Can you work these out from the model? Positions are in its coordinate system, mm. A direction names the side the tool comes from. Give positions to 0.01 mm unless a question says otherwise; leave off trailing zeros. Order: outer loops, then holes, each group sorted by start corner. A loop starts at its lowest first (then second) coordinate and runs counter-clockwise, first axis right, second up. Notation, with made-up numbers: (-29, 18) - (-5, 18) arc R21 cw to (-5, 40) - close; hole circle Ø3 at (16, 89.5). An arc over 180 degrees is marked (long way). Use one line per item in the form item = value. Start each with the question number.
1) Suppose I cut it at D-D, the plane z = 34.5. Write out the boundary of the cut face in (x, y).
2) Which directions (+Z, -Z, +X, -X, +Y, -Y) give clear straight access to the entire face, cutting with the end or side of a thin tool? Please do faces 5 (the flat face through (3, -1, 14)), 6 (the flat face through (7, 30, 1)), 7 (the flat face through (14, 0, 26)), 8 (the flat face through (14, -2, 1)), 9 (the flat face through (15, -22, 36)).
3) Suppose I cut it at C-C, the plane x = 5.25. Write out the boundary of the cut face in (y, z).
4) Please list where these lines run through material, in increasing order: probe 1 along Y at (x, z) = (24.75, 1.1); probe 2 along X at (y, z) = (-1, 23); probe 3 along Y at (x, z) = (26.25, 36).
5) We'd pull the mould along Z, two halves only. Please class faces 1 (the flat face through (15, 19, 0)), 2 (the flat face through (23, 30, 1)), 3 (the flat face through (15, -21, 47)), 4 (the cylindrical face through (9.1, -21, 35.7)): released by +Z, released by -Z, zero draft, split by the parting line, or undercut.
6) Suppose I cut it at A-A, the plane x = 10. Write out the boundary of the cut face in (y, z), and give its area (4 significant figures).
7) For pin 1 (1.8 mm diameter, centred on x = 20, z = 34.5, fed in from +Y); pin 2 (4 mm diameter, centred on x = 9, y = 5, fed in from +Z); pin 3 (17.5 mm diameter, centred on x = 12, y = -12.5, fed in from -Z); pin 4 (0.6 mm diameter, centred on x = 17, z = 1.5, fed in from -Y), each with a flat end and sliding along its axis, tell me the tip position at first contact or that it passes through.
8) Suppose I cut it at B-B, the plane z = 9. Write out the boundary of the cut face in (x, y), and give its area (3 significant figures).
```python
from build123d import *

# Parameters (mm, degrees)
SKETCH1_W           = 30
SKETCH1_H           = 40
BOSS_EXTRUDE1_DEPTH = 2
BOSS_EXTRUDE3_DEPTH = 30
SKETCH6_W           = 24
SKETCH6_H           = 23
CUT_EXTRUDE2_DEPTH  = 2
SKETCH7_R           = 1.5
SKETCH7_W           = 16
SKETCH7_H           = 2.75
CUT_EXTRUDE3_DEPTH  = 10
SKETCH9_R           = 1.5
CUT_EXTRUDE4_DEPTH  = 10


with BuildPart() as part:
    # Sketch1 → Boss-Extrude1 (new body)
    with BuildSketch(Plane.XY):
        with Locations((15, 20)):
            Rectangle(SKETCH1_W, SKETCH1_H)
    extrude(amount=BOSS_EXTRUDE1_DEPTH)

    # Sketch5 → Boss-Extrude3 (add)
    with BuildSketch(Plane(origin=(0, 0, 0), x_dir=(0, 0, -1), z_dir=(1, 0, 0))):
        Polygon((-27, -20), (-47, -20), (-47, -22), (-26.3, -22), (-25, -22), (-25, -2), (0, -2), (0, 0), (-2, 0), (-27, 0), align=None)
    extrude(amount=BOSS_EXTRUDE3_DEPTH)

    # Sketch6 → Cut-Extrude2 (cut)
    with BuildSketch(Plane(origin=(0, 0, 0), x_dir=(1, 0, 0), z_dir=(0, 1, 0))):
        with Locations((15, -13.5)):
            Rectangle(SKETCH6_W, SKETCH6_H)
    extrude(amount=-CUT_EXTRUDE2_DEPTH, mode=Mode.SUBTRACT)

    # Sketch7 → Cut-Extrude3 (cut)
    with BuildSketch(Plane(origin=(0, 0, 0), x_dir=(-1, 0, 0), z_dir=(0, 0, -1))):
        with Locations((-24.75, 25.797552116)):
            Circle(SKETCH7_R)
        with Locations((-5.25, 25.797552116)):
            Circle(SKETCH7_R)
        with Locations((-15, 29.922552116)):
            Rectangle(SKETCH7_W, SKETCH7_H)
    extrude(amount=-CUT_EXTRUDE3_DEPTH, mode=Mode.SUBTRACT)

    # Sketch9 → Cut-Extrude4 (cut)
    with BuildSketch(Plane.XZ.offset(22)):
        with Locations(Location((20, 34.5, 0), (0, 0, 270))):
            Circle(SKETCH9_R)
        with Locations(Location((10, 34.5, 0), (0, 0, 270))):
            Circle(SKETCH9_R)
    extrude(amount=-CUT_EXTRUDE4_DEPTH, mode=Mode.SUBTRACT)


solid = part.part
```
Result sheet:
q1.outline = (0, -22) - (8.5, -22) - (8.5, -20) - (0, -20) - close; (11.5, -22) - (18.5, -22) - (18.5, -20) - (11.5, -20) - close; (21.5, -22) - (30, -22) - (30, -20) - (21.5, -20) - close
q2.face_5 = +Y, -Y
q2.face_6 = +Z, -Z
q2.face_7 = +Z, +X, -X, +Y
q2.face_8 = -Z, +X, -X, -Y
q2.face_9 = +Z, -Z, +X, -X, -Y
q3.outline = (-22, 25) - (0, 25) - (0, 27) - (-20, 27) - (-20, 47) - (-22, 47) - close; (-2, 0) - (24.3, 0) - (24.3, 2) - (-2, 2) - close; (27.3, 0) - (40, 0) - (40, 2) - (27.3, 2) - close
q4.probe_1 = -2 to 24.3, 27.3 to 40
q4.probe_2 = 0 to 3, 27 to 30
q4.probe_3 = -22 to -20
q5.face_1 = released by -Z
q5.face_2 = zero draft
q5.face_3 = released by +Z
q5.face_4 = undercut
q6.outline = (-22, 25) - (0, 25) - (0, 27) - (-20, 27) - (-20, 33) - (-22, 33) - close; (-22, 36) - (-20, 36) - (-20, 47) - (-22, 47) - close; (-2, 0) - (28.55, 0) - (28.55, 2) - (-2, 2) - close; (31.3, 0) - (40, 0) - (40, 2) - (31.3, 2) - close
q6.area = 156.5 mm²
q7.pin_1 = through
q7.pin_2 = 2
q7.pin_3 = 25
q7.pin_4 = -2
q8.outline = (0, -2) - (3, -2) - (3, 0) - (0, 0) - close; (27, -2) - (30, -2) - (30, 0) - (27, 0) - close
q8.area = 12.0 mm²
